```python
from build123d import *

# Parameters (mm, degrees)
SKETCH1_W                = 5
SKETCH1_H                = 2
BOSS_EXTRUDE1_DEPTH      = 2
SKETCH2_W                = 4
SKETCH2_H                = 0.75
CUT_EXTRUDE1_DEPTH       = 6.744562647
CHAMFER1_START           = -1.060660172
CHAMFER1_OUTLINE_W       = 1.403805922
CHAMFER1_OUTLINE_H       = 3
CHAMFER1_OUTLINE_W_2     = 1.353553391
CHAMFER1_DEPTH           = 4.242640687
CHAMFER1_START_2         = 3.181980515
CHAMFER1_2_OUTLINE_W     = 4.242640687
CHAMFER1_2_OUTLINE_H     = 3
CHAMFER1_2_DEPTH         = 1.818019485
CHAMFER1_START_3         = -1.414213562
CHAMFER1_3_OUTLINE_W     = 4.242640687
CHAMFER1_3_OUTLINE_H     = 3
CHAMFER1_3_DEPTH         = 0.35355339
BOSS_EXTRUDE2_DEPTH      = 5
BOSS_EXTRUDE2_DEPTH_BACK = 5
SKETCH3_W                = 0.5
SKETCH3_H                = 0.5


with BuildPart() as part:
    # Sketch1 → Boss-Extrude1 (new body)
    with BuildSketch(Plane(origin=(0, 0, 0), x_dir=(1, 0, 0), z_dir=(0, 1, 0))):
        with Locations((2.5, 1)):
            Rectangle(SKETCH1_W, SKETCH1_H)
    extrude(amount=BOSS_EXTRUDE1_DEPTH)

    # Sketch2 → Cut-Extrude1 (cut, through all)
    with BuildSketch(Plane.XY):
        with Locations((2.5, 0.375)):
            Rectangle(SKETCH2_W, SKETCH2_H)
    extrude(amount=-CUT_EXTRUDE1_DEPTH, mode=Mode.SUBTRACT)

    # Chamfer1: read off the stored shape, not the designer's step
    # Chamfer1 outline → Chamfer1 (cut)
    with BuildSketch(Plane(origin=(0, 0, 0), x_dir=(0.707106781186549, 0, -0.707106781186546), z_dir=(0.707106781186546, 0, 0.707106781186549)).offset(CHAMFER1_START)):
        with Locations((5.298097039, 1.5)):
            Rectangle(CHAMFER1_OUTLINE_W, CHAMFER1_OUTLINE_H)
        with Locations((-0.323223305, 1.5)):
            Rectangle(CHAMFER1_OUTLINE_W_2, CHAMFER1_OUTLINE_H)
    extrude(amount=CHAMFER1_DEPTH, mode=Mode.SUBTRACT)

    # Chamfer1 2 outline → Chamfer1 2 (cut)
    with BuildSketch(Plane(origin=(0, 0, 0), x_dir=(0.707106781186549, 0, -0.707106781186546), z_dir=(0.707106781186546, 0, 0.707106781186549)).offset(CHAMFER1_START_2)):
        with Locations((2.474873735, 1.5)):
            Rectangle(CHAMFER1_2_OUTLINE_W, CHAMFER1_2_OUTLINE_H)
    extrude(amount=CHAMFER1_2_DEPTH, mode=Mode.SUBTRACT)

    # Chamfer1 3 outline → Chamfer1 3 (cut)
    with BuildSketch(Plane(origin=(0, 0, 0), x_dir=(0.707106781186549, 0, -0.707106781186546), z_dir=(0.707106781186546, 0, 0.707106781186549)).offset(CHAMFER1_START_3)):
        with Locations((2.474873735, 1.5)):
            Rectangle(CHAMFER1_3_OUTLINE_W, CHAMFER1_3_OUTLINE_H)
    extrude(amount=CHAMFER1_3_DEPTH, mode=Mode.SUBTRACT)

    # Sketch3 → Boss-Extrude2 (add, two sides: drawn at the far end of the back side and taken through both)
    with BuildSketch(Plane(origin=(0, 2, 0), x_dir=(1, 0, 0), z_dir=(0, 1, 0)).offset(-BOSS_EXTRUDE2_DEPTH_BACK)):
        with Locations((1.25, 1)):
            Rectangle(SKETCH3_W, SKETCH3_H)
        with Locations((3.75, 1)):
            Rectangle(SKETCH3_W, SKETCH3_H)
    extrude(amount=BOSS_EXTRUDE2_DEPTH + BOSS_EXTRUDE2_DEPTH_BACK)


solid = part.part
```
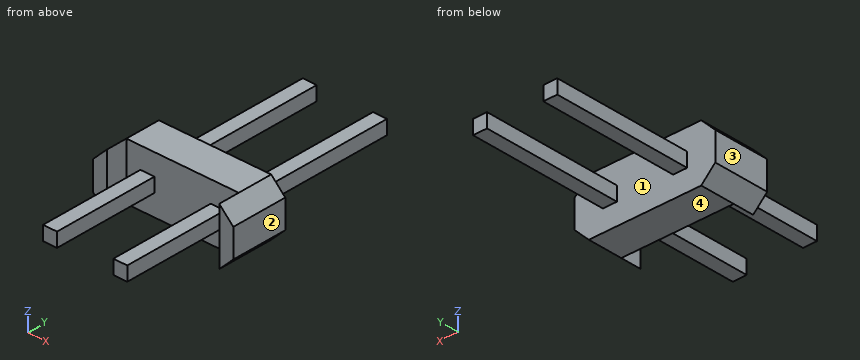
Here's how the part is built. I have some questions about the finished solid (model axes, mm). Face numbers are marked on the shaded views. Give positions to 0.01 mm unless a question says otherwise; leave off trailing zeros. Order: outer loops, then holes, each group sorted by start corner. A loop starts at its lowest first (then second) coordinate and runs counter-clockwise, first axis right, second up. Notation, with made-up numbers: M 88,-33 L 107,-33 A15 cw 107,-12 Z; hole C -19.75,67 d7. An arc over 180 degrees is marked long. Use a Markdown table: item, result. Add a question column.
1. If we mould it in two halves opening along X, with no side actions, what happens to the marked faces 1, 2, 3 and 4? For each: +X half, -X half, draft (parallel to the pull), parting line (faces both ways), or undercut.
2. Suppose I cut it at D-D (x = 3.9). List the corners of the cut face in (y, z) for me.
3. Suppose I cut it at A-A (y = 4.5). List the corners of the cut face in (x, z) for me, and give its area (3 significant figures).
4. I need wall thicknesses on probe 1 along X at (y, z) = (2.5, -0.8); probe 2 along Y at (x, z) = (2.4, -1.45); probe 3 along X at (y, z) = (0.25, -0.6). Which ranges of each line are inside material? Lowest first, please. Write a range as from..to.
5. Suppose I cut it at C-C (y = 1). List the corners of the cut face in (x, z) for me, and give its area (3 significant figures).
6. Suppose I cut it at B-B (z = -0.3). List the corners of the cut face in (x, y) for me, and give its area (3 significant figures).
7. For pin 1 Ø1 at (y, z) = (-1, -1.5) entering from -X; pin 2 Ø1.5 at (x, y) = (1, 5) entering from -Z; pin 3 Ø0.6 at (x, z) = (2.5, -1.5) entering from -Y, each with a flat end and sliding along its axis, tell me the tip position at first contact or that it passes through.
Results list:
| question | item | result |
|---|---|---|
| 1 | face 1 | undercut |
| 1 | face 2 | +X half |
| 1 | face 3 | -X half |
| 1 | face 4 | draft |
| 2 | outline | M -3,-1.25 L 0.75,-1.25 L 0.75,-2 L 2,-2 L 2,-1.25 L 7,-1.25 L 7,-0.75 L 2,-0.75 L 2,0 L 0.75,0 L 0.75,-0.75 L -3,-0.75 Z |
| 3 | outline | M 1,-1.25 L 1.5,-1.25 L 1.5,-0.75 L 1,-0.75 Z; M 3.5,-1.25 L 4,-1.25 L 4,-0.75 L 3.5,-0.75 Z |
| 3 | area | 0.500 mm² |
| 4 | probe 1 | x = 1..1.5, 3.5..4 |
| 4 | probe 2 | y = 0.75..2 |
| 4 | probe 3 | x = 0..0.5, 4.5..5 |
| 5 | outline | M 0,-1.5 L 0.5,-2 L 4.5,-2 L 5,-1.5 L 5,-0.5 L 4.5,0 L 0.5,0 L 0,-0.5 Z |
| 5 | area | 9.50 mm² |
| 6 | outline | M 0.2,0 L 0.5,0 L 0.5,0.75 L 4.5,0.75 L 4.5,0 L 4.8,0 L 4.8,2 L 0.2,2 Z |
| 6 | area | 6.20 mm² |
| 7 | pin 1 | stops at x = 1 |
| 7 | pin 2 | stops at z = -1.25 |
| 7 | pin 3 | stops at y = 0.75 |
